```python
from build123d import *

# Parameters (mm, degrees)
BASE_FLANGE3_DEPTH        = 100
SKETCH16_R                = 18
CUT_EXTRUDE1_DEPTH        = 10
F_4_0MM_DOWEL_HOLE1_D     = 4
F_5_0MM_DOWEL_HOLE1_D     = 5
F_5_0MM_DOWEL_HOLE1_DEPTH = 98.31
F_5_0MM_DOWEL_HOLE1_TIP   = 1.502151548


# Sheet-metal steps are written as plain solids
with BuildPart() as part:
    # Sketch1 → Base-Flange3 (new body)
    with BuildSketch(Plane.XY):
        with BuildLine():
            Line((110, 0), (2, 0))
            ThreePointArc((2, 0), (0.585786438, -0.585786438), (0, -2))
            Line((0, -2), (0, -88))
            ThreePointArc((0, -88), (0.585786438, -89.414213562), (2, -90))
            Line((2, -90), (110, -90))
            Line((110, -90), (110, -94))
            Line((110, -94), (2, -94))
            ThreePointArc((2, -94), (-2.242640687, -92.242640687), (-4, -88))
            Line((-4, -88), (-4, -2))
            ThreePointArc((-4, -2), (-2.242640687, 2.242640687), (2, 4))
            Line((2, 4), (110, 4))
            Line((110, 4), (110, 0))
        make_face()
    extrude(amount=BASE_FLANGE3_DEPTH)

    # Sketch16 → Cut-Extrude1 (cut)
    with BuildSketch(Plane.ZY.offset(4)):
        with Locations((50, -45.153641777)):
            Circle(SKETCH16_R)
    extrude(amount=-CUT_EXTRUDE1_DEPTH, mode=Mode.SUBTRACT)

    # Ø4.0mm Dowel Hole1 (through all)
    with Locations(Plane(origin=(0, -94, 0), x_dir=(-1, 0, 0), z_dir=(0, -1, 0))):
        with Locations((-32, -86.483109463), (-32, -13.516890537), (-88.463106056, -86.483109463), (-88.463106056, -13.516890537)):
            Hole(F_4_0MM_DOWEL_HOLE1_D / 2)

    # Ø5.0mm Dowel Hole1
    with Locations(Plane.ZY.offset(4)):
        with Locations((50, -10.153641777), (85, -45.153641777), (50, -80.153641777), (15, -45.153641777)):
            Hole(F_5_0MM_DOWEL_HOLE1_D / 2, depth=F_5_0MM_DOWEL_HOLE1_DEPTH)
            with Locations((0, 0, -(F_5_0MM_DOWEL_HOLE1_DEPTH + F_5_0MM_DOWEL_HOLE1_TIP / 2))):  # 118° drill point
                Cone(0, F_5_0MM_DOWEL_HOLE1_D / 2, F_5_0MM_DOWEL_HOLE1_TIP, mode=Mode.SUBTRACT)


solid = part.part
```
Could you check a few things on this model? Use its own coordinates, in mm. A direction names the side the tool comes from. Round coordinates to 2 decimals unless told otherwise and drop trailing zeros. Write each loop counter-clockwise with the first axis right and the second up, starting at its lowest first coordinate (ties: lowest second). Pieces come first, ordered by that corner, then holes.
(1) Which directions (+Z, -Z, +X, -X, +Y, -Y) give clear straight access to the entire face, cutting with the end or side of a thin tool? Please do faces 4 (the face through (57, -94, 49)), 5 (the face through (57, 0, 49)).
Findings below:
face 4: +Z, -Z, +X, -X, -Y
face 5: +Z, -Z, +X
(2) Suppose I cut it at C-C on x = 32. Write out the boundary of the cut face in (y, z).
Findings below:
outline: (-94, 0) - (-90, 0) - (-90, 11.52) - (-94, 11.52) - close; (-94, 15.52) - (-90, 15.52) - (-90, 84.48) - (-94, 84.48) - close; (-94, 88.48) - (-90, 88.48) - (-90, 100) - (-94, 100) - close; (0, 0) - (4, 0) - (4, 11.52) - (0, 11.52) - close; (0, 15.52) - (4, 15.52) - (4, 84.48) - (0, 84.48) - close; (0, 88.48) - (4, 88.48) - (4, 100) - (0, 100) - close
(3) Thinking about a two-plate mould opening in X: for faces 1 (the face through (55, 4, 49)), 2 (the face through (33.85, -91.97, 14.28)), 3 (the face through (-2.196, -92.289, 49.3)), which applies, +X half, -X half, draft (parallel to the pull), parting line (faces both ways), or undercut?
Findings below:
face 1: draft
face 2: undercut
face 3: -X half
(4) For pin 1 (4 mm diameter, centred on y = -80.15, z = 50, fed in from +X); pin 2 (8 mm diameter, centred on y = -31.5, z = 23, fed in from +X), each with a flat end and sliding along its axis, tell me the tip position at first contact or that it passes through.
Findings below:
pin 1: passes through
pin 2: stops at x = 0
(5) If I drill on probe 1 along Z at (x, y) = (32, 0.95); probe 2 along Y at (x, z) = (65.5, 83); probe 3 along X at (y, z) = (-69.5, 15), over which ranges is the centre line in solid material (lowest first)?
Findings below:
probe 1: z = 0 to 11.52, 15.52 to 84.48, 88.48 to 100
probe 2: y = -94 to -90, 0 to 4
probe 3: x = -4 to 0
(6) Suppose I cut it at D-D on z = 33.5. Write out the boundary of the cut face in (x, y), and give its area (3 significant figures).
Findings below:
outline: (-4, -88) arc R6 ccw to (2, -94) - (110, -94) - (110, -90) - (2, -90) arc R2 cw to (0, -88) - (0, -52.35) - (-4, -52.35) - close; (-4, -37.96) - (0, -37.96) - (0, -2) arc R2 cw to (2, 0) - (110, 0) - (110, 4) - (2, 4) arc R6 ccw to (-4, -2) - close
area: 1,200 mm2
(7) Suppose I cut it at A-A on x = 46.5. Write out the boundary of the cut face in (y, z).
Findings below:
outline: (-94, 0) - (-90, 0) - (-90, 100) - (-94, 100) - close; (0, 0) - (4, 0) - (4, 100) - (0, 100) - close
(8) Suppose I cut it at B-B on z = 50. Write out the boundary of the cut face in (x, y), and give its area (3 significant figures).
Findings below:
outline: (-4, -88) arc R6 ccw to (2, -94) - (110, -94) - (110, -90) - (2, -90) arc R2 cw to (0, -88) - (0, -82.65) - (-4, -82.65) - close; (-4, -77.65) - (0, -77.65) - (0, -63.15) - (-4, -63.15) - close; (-4, -27.15) - (0, -27.15) - (0, -12.65) - (-4, -12.65) - close; (-4, -7.65) - (0, -7.65) - (0, -2) arc R2 cw to (2, 0) - (110, 0) - (110, 4) - (2, 4) arc R6 ccw to (-4, -2) - close
area: 1,070 mm2
